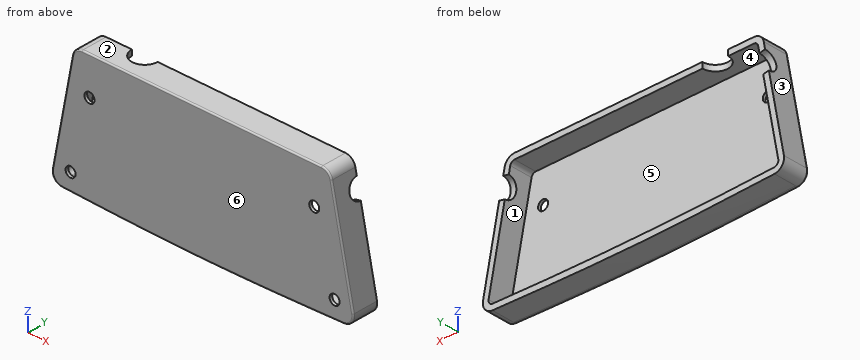
from build123d import *

# Parameters (mm, degrees)
SKETCH1_R           = 1.75
BOSS_EXTRUDE1_DEPTH = 1
BOSS_EXTRUDE2_DEPTH = 9
CUT_EXTRUDE2_DEPTH  = 2
CUT_EXTRUDE3_DEPTH  = 7
FILLET1_R           = 0.5
CUT_EXTRUDE4_DEPTH  = 2


with BuildPart() as part:
    # Sketch1 → Boss-Extrude1 (new body)
    with BuildSketch(Plane(origin=(0, 0, 0), x_dir=(1, 0, 0), z_dir=(0, 1, 0))):
        with BuildLine():
            ThreePointArc((-3.131484069, 5.892071798), (-5.737365292, 4.575348005), (-6.438282309, 1.7410767))
            Line((-6.438282309, 1.7410767), (0.60003894, -35.29332564))
            ThreePointArc((0.60003894, -35.29332564), (1.806583814, -37.335883181), (4.03849413, -38.139853444))
            Line((4.03849413, -38.139853444), (87.670939293, -38.139853444))
            ThreePointArc((87.670939293, -38.139853444), (89.884160785, -37.35124619), (91.100032265, -35.340796659))
            Line((91.100032265, -35.340796659), (98.669943789, 1.692061139))
            ThreePointArc((98.669943789, 1.692061139), (97.993413035, 4.554809441), (95.372557333, 5.890525389))
            add(Edge.make_bspline(
                [(-3.131484069, 5.892071798), (46.109282616, 7.745637681), (95.372557333, 5.890525389)],
                knots=[0.096020277, 0.096020277, 0.096020277, 0.904206285, 0.904206285, 0.904206285], degree=2, weights=[1.148800657, 1.708499103, 1.148486764]))
        make_face()
        with BuildLine():
            ThreePointArc((95.297296467, 3.89194194), (96.420520339, 3.319492248), (96.710462091, 2.092600119))
            Line((96.710462091, 2.092600119), (89.140550566, -34.940257679))
            ThreePointArc((89.140550566, -34.940257679), (88.619462789, -35.801878907), (87.670939293, -36.139853444))
            Line((87.670939293, -36.139853444), (4.03849413, -36.139853444))
            ThreePointArc((4.03849413, -36.139853444), (3.081961137, -35.79529476), (2.564870477, -34.919912956))
            Line((2.564870477, -34.919912956), (-4.473450772, 2.114489384))
            ThreePointArc((-4.473450772, 2.114489384), (-4.173057765, 3.329177086), (-3.056251526, 3.893487283))
            ThreePointArc((-3.056251526, 3.893487283), (46.120537007, 4.817927579), (95.297296467, 3.89194194))
        make_face(mode=Mode.SUBTRACT)
        with BuildLine():
            Line((89.140550566, -34.940257679), (96.710462091, 2.092600119))
            ThreePointArc((96.710462091, 2.092600119), (96.420520339, 3.319492248), (95.297296467, 3.89194194))
            ThreePointArc((95.297296467, 3.89194194), (46.120537007, 4.817927579), (-3.056251526, 3.893487283))
            ThreePointArc((-3.056251526, 3.893487283), (-4.173057765, 3.329177086), (-4.473450772, 2.114489384))
            Line((-4.473450772, 2.114489384), (2.564870477, -34.919912956))
            ThreePointArc((2.564870477, -34.919912956), (3.081961137, -35.79529476), (4.03849413, -36.139853444))
            Line((4.03849413, -36.139853444), (87.670939293, -36.139853444))
            ThreePointArc((87.670939293, -36.139853444), (88.619462789, -35.801878907), (89.140550566, -34.940257679))
        make_face()
        with Locations((6.60003894, -24.999988489)):
            Circle(SKETCH1_R, mode=Mode.SUBTRACT)
        with Locations((85.100032265, -24.999862922)):
            Circle(SKETCH1_R, mode=Mode.SUBTRACT)
        Circle(SKETCH1_R, mode=Mode.SUBTRACT)
        with Locations((92.2, 0)):
            Circle(SKETCH1_R, mode=Mode.SUBTRACT)
    extrude(amount=BOSS_EXTRUDE1_DEPTH)

    # Sketch1_5 → Boss-Extrude2 (add)
    with BuildSketch(Plane(origin=(0, 0, 0), x_dir=(1, 0, 0), z_dir=(0, 1, 0))):
        with BuildLine():
            ThreePointArc((-3.131484069, 5.892071798), (-5.737365292, 4.575348005), (-6.438282309, 1.7410767))
            Line((-6.438282309, 1.7410767), (0.60003894, -35.29332564))
            ThreePointArc((0.60003894, -35.29332564), (1.806583814, -37.335883181), (4.03849413, -38.139853444))
            Line((4.03849413, -38.139853444), (87.670939293, -38.139853444))
            ThreePointArc((87.670939293, -38.139853444), (89.884160785, -37.35124619), (91.100032265, -35.340796659))
            Line((91.100032265, -35.340796659), (98.669943789, 1.692061139))
            ThreePointArc((98.669943789, 1.692061139), (97.993413035, 4.554809441), (95.372557333, 5.890525389))
            add(Edge.make_bspline(
                [(-3.131484069, 5.892071798), (46.109282616, 7.745637681), (95.372557333, 5.890525389)],
                knots=[0.096020277, 0.096020277, 0.096020277, 0.904206285, 0.904206285, 0.904206285], degree=2, weights=[1.148800657, 1.708499103, 1.148486764]))
        make_face()
        with BuildLine():
            ThreePointArc((95.297296467, 3.89194194), (96.420520339, 3.319492248), (96.710462091, 2.092600119))
            Line((96.710462091, 2.092600119), (89.140550566, -34.940257679))
            ThreePointArc((89.140550566, -34.940257679), (88.619462789, -35.801878907), (87.670939293, -36.139853444))
            Line((87.670939293, -36.139853444), (4.03849413, -36.139853444))
            ThreePointArc((4.03849413, -36.139853444), (3.081961137, -35.79529476), (2.564870477, -34.919912956))
            Line((2.564870477, -34.919912956), (-4.473450772, 2.114489384))
            ThreePointArc((-4.473450772, 2.114489384), (-4.173057765, 3.329177086), (-3.056251526, 3.893487283))
            ThreePointArc((-3.056251526, 3.893487283), (46.120537007, 4.817927579), (95.297296467, 3.89194194))
        make_face(mode=Mode.SUBTRACT)
    extrude(amount=BOSS_EXTRUDE2_DEPTH)

    # Sketch2 → Cut-Extrude2 (cut)
    with BuildSketch(Plane(origin=(94.380499607, 0, 19.292381797), x_dir=(0.20026949, 0, -0.979740849), z_dir=(0.979740849, 0, 0.20026949))):
        with BuildLine():
            Line((-6.880265125, 9), (-13.880265125, 9))
            ThreePointArc((-13.880265125, 9), (-10.380265125, 5.5), (-6.880265125, 9))
        make_face()
    extrude(amount=-CUT_EXTRUDE2_DEPTH, mode=Mode.SUBTRACT)

    # Sketch3 → Cut-Extrude3 (cut)
    with BuildSketch(Plane.XY.offset(38.139853444)):
        with BuildLine():
            Line((22.03849413, 9), (13.03849413, 9))
            ThreePointArc((13.03849413, 9), (17.53849413, 4.5), (22.03849413, 9))
        make_face()
    extrude(amount=-CUT_EXTRUDE3_DEPTH, mode=Mode.SUBTRACT)

    # Fillet1
    fillet1_edges = [part.edges().sort_by_distance(p)[0] for p in [
        (97.993413035, 0, -4.554809441),
        (94.884988027, 0, 16.82436776),
        (89.884160785, 0, 37.35124619),
        (45.854716711, 0, 38.139853444),
        (1.806583814, 0, 37.335883181),
        (-2.919121684, 0, 16.77612447),
        (-5.737365292, 0, -4.575348005),
        (46.120186786, 0, -7.000146325),
    ]]
    fillet(fillet1_edges, radius=FILLET1_R)

    # Sketch4 → Cut-Extrude4 (cut)
    with BuildSketch(Plane(origin=(-5.89449461, 0, 1.12023805), x_dir=(0.186706342, 0, 0.982415768), z_dir=(-0.982415768, 0, 0.186706342))):
        with BuildLine():
            Line((25.284750703, 9), (32.284750703, 9))
            ThreePointArc((32.284750703, 9), (28.784750703, 5.5), (25.284750703, 9))
        make_face()
    extrude(amount=-CUT_EXTRUDE4_DEPTH, mode=Mode.SUBTRACT)


solid = part.part
Input: part model. Units: mm. Frame: model coordinates. Face numbers are marked on the shaded views. A direction names the side the tool comes from. Coordinates: 2 decimals unless noted, no trailing zeros. Answer in a Markdown table with one row per item. Add a question column.
Item 1: Mould query, pull axis Z, two halves, no side actions, for the marked faces 3, 4, 5 and 6. Classes: released by +Z, released by -Z, zero draft, split by the parting line, or undercut.
Item 2: Line query: line 1 along X through (y, z) = (0.6, 0); line 2 along Y through (x, z) = (33, -2); line 3 along X through (y, z) = (6.5, -1.5). Output: solid intervals per line, ascending. Write a range as [from, to].
Item 3: Access query for the marked faces 1 and 2. Directions: +Z, -Z, +X, -X, +Y, -Y. A direction counts if a zero-diameter tool reaches every point of the face in a straight line with its end or side. Return the directions, or none.
Item 4: Section query A-A on y = 7.5. State how many separate pieces and enclosed holes the cut face has, then the cut area to 3 significant figures.
Item 5: Contact query for flat-ended pins moving along their axis: P1, Ø10, axis at x = 38.5, z = 29, coming from the +Y side; P2, Ø4, axis at y = 4, z = 23, coming from the +X side; P3, Ø1, axis at x = 81, y = 2, coming from the -Z side; P4, Ø4, axis at x = 47.5, y = 7, coming from the -Z side. Output: stop coordinate, or through.
Recorded:
| question | item | result |
|---|---|---|
| 1 | face 3 | released by +Z |
| 1 | face 4 | undercut |
| 1 | face 5 | undercut |
| 1 | face 6 | zero draft |
| 2 | line 1 | [-6.11, -1.75], [1.75, 90.45], [93.95, 98.32] |
| 2 | line 2 | [0, 1] |
| 2 | line 3 | [-6.39, -4.36], [96.59, 98.63] |
| 3 | face 1 | +Y |
| 3 | face 2 | +Z, +X, -X, +Y, -Y |
| 4 | separate pieces | 3 |
| 4 | enclosed holes | 0 |
| 4 | area | 513 mm^2 |
| 5 | P1 | y = 1 |
| 5 | P2 | x = 94.03 |
| 5 | P3 | z = -6.41 |
| 5 | P4 | z = -7 |
